Here's how the part is built. I have some questions about the finished solid (model axes, mm). A direction names the side the tool comes from. Give positions to 0.01 mm unless a question says otherwise; leave off trailing zeros. Order: outer loops, then holes, each group sorted by start corner. A loop starts at its lowest first (then second) coordinate and runs counter-clockwise, first axis right, second up. Notation, with made-up numbers: M 42,-19.75 L 66,-19.75 A19 ccw 66,0.25 Z; hole C 67,77 d11. An arc over 180 degrees is marked long. Use one line per item in the form item = value.
from build123d import *

# Parameters (mm, degrees)
F1_DEPTH  = 5
F0_W      = 15
F0_H      = 3
F2_DEPTH  = 15
F0_W_2    = 3
F3_DEPTH  = 3
F4_DEPTH  = 12
F6_DEPTH  = 25
F10_W     = 5
F10_H     = 5
F11_DEPTH = 2
F12_DEPTH = 12
F13_DEPTH = 9
F14_DEPTH = 6
F15_DEPTH = 9
F16_DEPTH = 9
F17_DEPTH = 15
F18_DEPTH = 12
F19_DEPTH = 6
F20_DEPTH = 9
F21_DEPTH = 12
F22_DEPTH = 9
F23_DEPTH = 3
F24_DEPTH = 4
F25_DEPTH = 6
F26_DEPTH = 1
F27_DEPTH = 3
F28_DEPTH = 5
F9_W      = 3
F9_H      = 3
F29_DEPTH = 2
F30_DEPTH = 4
F31_DEPTH = 6
F32_DEPTH = 8
F33_DEPTH = 1
F34_DEPTH = 3
F35_DEPTH = 5
F36_DEPTH = 7
F37_DEPTH = 1
F38_DEPTH = 2
F39_DEPTH = 3
F40_DEPTH = 4
F42_DEPTH = 3
F44_DEPTH = 3


with BuildPart() as f1:
    # F0 (on Top) → F1 (new body)
    with BuildSketch(Plane.XY):
        Polygon((14.2212225916, -3.3255452978), (14.1498658388, 11.6744547022), (-0.7787774084, 11.6744547022), (-0.7787774084, -3.3255452978), align=None)
    extrude(amount=F1_DEPTH)



with BuildPart() as f2:
    # F0 (on Top) → F2 (new body)
    with BuildSketch(Plane.XY):
        with Locations((-11.4361313693, -1.8255452978)):
            Rectangle(F0_W, F0_H)
    extrude(amount=F2_DEPTH)


with BuildPart() as f3:
    # F0 (on Top) → F3 (new body)
    with BuildSketch(Plane.XY):
        with Locations((-5.4361313693, 28.1744547022)):
            Rectangle(F0_W_2, F0_H)
    extrude(amount=F3_DEPTH)


with BuildPart() as f4:
    # F0 (on Top) → F4 (new body)
    with BuildSketch(Plane.XY):
        Polygon((2.0638686307, 29.6744547022), (-0.9361313693, 29.6744547022), (-0.9361313693, 14.7520447022), (-0.9361313693, 14.6744547022), (2.0638686307, 14.6744547022), (2.0638686307, 14.7520447022), align=None)
    extrude(amount=F4_DEPTH)


with BuildPart() as f1_1:
    add(f1.part)

    add(f2.part)  # F6 merges F2

    add(f3.part)  # F6 merges F3

    add(f4.part)  # F6 merges F4
    # F5 (on Top) → F6 (join)
    with BuildSketch(Plane.XY):
        Polygon((-18.9361313693, -3.3255452978), (14.2212225916, -3.3255452978), (14.0638686307, 29.7520447022), (-18.9361313693, 29.6744547022), align=None)
    extrude(amount=-F6_DEPTH)

    # F7 (on face) → F8 (revolve, cut)
    with BuildSketch(Plane.XZ.offset(3.3255452978)):
        with BuildLine():
            Line((-2.1231973078, -23.52852803), (-2.1231973078, -2.4096941548))
            ThreePointArc((-2.1231973078, -2.4096941548), (-12.6826142454, -12.9691110924), (-2.1231973078, -23.52852803))
        make_face()
    revolve(axis=Axis((-2.1231973078, -3.3255452978, -12.9691110924), (0, 0, -1)), mode=Mode.SUBTRACT)

    # F10 (on face) → F11 (cut)
    with BuildSketch(Plane(origin=(14.2050811207, 0.0675752308, 0), x_dir=(-0.004757063, 0.9999886851, 0), z_dir=(0.9999886851, 0.004757063, 0))):
        with Locations((2.0033325977, -6.7919711024)):
            Rectangle(F10_W, F10_H)
    extrude(amount=-F11_DEPTH, mode=Mode.SUBTRACT)

    # F0 (on Top) → F12 (join)
    with BuildSketch(Plane.XY):
        with Locations((-11.4361313693, 4.1744547022)):
            Rectangle(F0_W, F0_H)
    extrude(amount=F12_DEPTH)

    # F0 (on Top) → F13 (join)
    with BuildSketch(Plane.XY):
        with Locations((-11.4361313693, 10.1744547022)):
            Rectangle(F0_W, F0_H)
    extrude(amount=F13_DEPTH)

    # F0 (on Top) → F14 (join)
    with BuildSketch(Plane.XY):
        with Locations((-11.4361313693, 28.1744547022)):
            Rectangle(F0_W_2, F0_H)
    extrude(amount=F14_DEPTH)

    # F0 (on Top) → F15 (join)
    with BuildSketch(Plane.XY):
        with Locations((-17.4361313693, 28.1744547022)):
            Rectangle(F0_W_2, F0_H)
    extrude(amount=F15_DEPTH)

    # F0 (on Top) → F16 (join)
    with BuildSketch(Plane.XY):
        with Locations((-11.4361313693, 22.1744547022)):
            Rectangle(F0_W_2, F0_H)
    extrude(amount=F16_DEPTH)

    # F0 (on Top) → F17 (join)
    with BuildSketch(Plane.XY):
        with Locations((-17.4361313693, 16.1744547022)):
            Rectangle(F0_W_2, F0_H)
    extrude(amount=F17_DEPTH)

    # F0 (on Top) → F18 (join)
    with BuildSketch(Plane.XY):
        with Locations((-17.4361313693, 22.1744547022)):
            Rectangle(F0_W_2, F0_H)
    extrude(amount=F18_DEPTH)

    # F0 (on Top) → F19 (join)
    with BuildSketch(Plane.XY):
        with Locations((-5.4361313693, 22.1744547022)):
            Rectangle(F0_W_2, F0_H)
    extrude(amount=F19_DEPTH)

    # F0 (on Top) → F20 (join)
    with BuildSketch(Plane.XY):
        with Locations((-5.4361313693, 16.1744547022)):
            Rectangle(F0_W_2, F0_H)
    extrude(amount=F20_DEPTH)

    # F0 (on Top) → F21 (join)
    with BuildSketch(Plane.XY):
        with Locations((-11.4361313693, 16.1744547022)):
            Rectangle(F0_W_2, F0_H)
    extrude(amount=F21_DEPTH)

    # F0 (on Top) → F22 (join)
    with BuildSketch(Plane.XY):
        Polygon((8.0638686307, 29.6744547022), (5.0638686307, 29.6744547022), (5.0638686307, 14.7520447022), (5.0638686307, 14.6744547022), (8.0638686307, 14.6744547022), (8.0638686307, 14.7520447022), align=None)
    extrude(amount=F22_DEPTH)

    # F0 (on Top) → F23 (join)
    with BuildSketch(Plane.XY):
        Polygon((14.0638686307, 29.6744547022), (11.0638686307, 29.6744547022), (11.0638686307, 14.7520447022), (11.0638686307, 14.6744547022), (14.0638686307, 14.6744547022), (14.0638686307, 14.7520447022), align=None)
    extrude(amount=F23_DEPTH)

    # F10 (on face) → F24 (cut)
    with BuildSketch(Plane(origin=(14.2050811207, 0.0675752308, 0), x_dir=(-0.004757063, 0.9999886851, 0), z_dir=(0.9999886851, 0.004757063, 0))):
        with Locations((12.0033325977, -6.7919711024)):
            Rectangle(F10_W, F10_H)
    extrude(amount=-F24_DEPTH, mode=Mode.SUBTRACT)

    # F10 (on face) → F25 (cut)
    with BuildSketch(Plane(origin=(14.2050811207, 0.0675752308, 0), x_dir=(-0.004757063, 0.9999886851, 0), z_dir=(0.9999886851, 0.004757063, 0))):
        with Locations((22.0033325977, -6.7919711024)):
            Rectangle(F10_W, F10_H)
    extrude(amount=-F25_DEPTH, mode=Mode.SUBTRACT)

    # F10 (on face) → F26 (cut)
    with BuildSketch(Plane(origin=(14.2050811207, 0.0675752308, 0), x_dir=(-0.004757063, 0.9999886851, 0), z_dir=(0.9999886851, 0.004757063, 0))):
        with Locations((2.0033325977, -16.7919711024)):
            Rectangle(F10_W, F10_H)
    extrude(amount=-F26_DEPTH, mode=Mode.SUBTRACT)

    # F10 (on face) → F27 (cut)
    with BuildSketch(Plane(origin=(14.2050811207, 0.0675752308, 0), x_dir=(-0.004757063, 0.9999886851, 0), z_dir=(0.9999886851, 0.004757063, 0))):
        with Locations((12.0033325977, -16.7919711024)):
            Rectangle(F10_W, F10_H)
    extrude(amount=-F27_DEPTH, mode=Mode.SUBTRACT)

    # F10 (on face) → F28 (cut)
    with BuildSketch(Plane(origin=(14.2050811207, 0.0675752308, 0), x_dir=(-0.004757063, 0.9999886851, 0), z_dir=(0.9999886851, 0.004757063, 0))):
        with Locations((22.0033325977, -16.7919711024)):
            Rectangle(F10_W, F10_H)
    extrude(amount=-F28_DEPTH, mode=Mode.SUBTRACT)

    # F9 (on face) → F29 (cut)
    with BuildSketch(Plane(origin=(-18.9361313693, 0, 0), x_dir=(0, -1, 0), z_dir=(-1, 0, 0))):
        with Locations((-23.521638004, -6.4509857927)):
            Rectangle(F9_W, F9_H)
    extrude(amount=-F29_DEPTH, mode=Mode.SUBTRACT)

    # F9 (on face) → F30 (cut)
    with BuildSketch(Plane(origin=(-18.9361313693, 0, 0), x_dir=(0, -1, 0), z_dir=(-1, 0, 0))):
        with Locations((-17.521638004, -6.4509857927)):
            Rectangle(F9_W, F9_H)
    extrude(amount=-F30_DEPTH, mode=Mode.SUBTRACT)

    # F9 (on face) → F31 (cut)
    with BuildSketch(Plane(origin=(-18.9361313693, 0, 0), x_dir=(0, -1, 0), z_dir=(-1, 0, 0))):
        with Locations((-11.521638004, -6.4509857927)):
            Rectangle(F9_W, F9_H)
    extrude(amount=-F31_DEPTH, mode=Mode.SUBTRACT)

    # F9 (on face) → F32 (cut)
    with BuildSketch(Plane(origin=(-18.9361313693, 0, 0), x_dir=(0, -1, 0), z_dir=(-1, 0, 0))):
        with Locations((-5.521638004, -6.4509857927)):
            Rectangle(F9_W, F9_H)
    extrude(amount=-F32_DEPTH, mode=Mode.SUBTRACT)

    # F9 (on face) → F33 (cut)
    with BuildSketch(Plane(origin=(-18.9361313693, 0, 0), x_dir=(0, -1, 0), z_dir=(-1, 0, 0))):
        with Locations((-23.521638004, -12.4509857927)):
            Rectangle(F9_W, F9_H)
    extrude(amount=-F33_DEPTH, mode=Mode.SUBTRACT)

    # F9 (on face) → F34 (cut)
    with BuildSketch(Plane(origin=(-18.9361313693, 0, 0), x_dir=(0, -1, 0), z_dir=(-1, 0, 0))):
        with Locations((-17.521638004, -12.4509857927)):
            Rectangle(F9_W, F9_H)
    extrude(amount=-F34_DEPTH, mode=Mode.SUBTRACT)

    # F9 (on face) → F35 (cut)
    with BuildSketch(Plane(origin=(-18.9361313693, 0, 0), x_dir=(0, -1, 0), z_dir=(-1, 0, 0))):
        with Locations((-11.521638004, -12.4509857927)):
            Rectangle(F9_W, F9_H)
    extrude(amount=-F35_DEPTH, mode=Mode.SUBTRACT)

    # F9 (on face) → F36 (cut)
    with BuildSketch(Plane(origin=(-18.9361313693, 0, 0), x_dir=(0, -1, 0), z_dir=(-1, 0, 0))):
        with Locations((-5.521638004, -12.4509857927)):
            Rectangle(F9_W, F9_H)
    extrude(amount=-F36_DEPTH, mode=Mode.SUBTRACT)

    # F9 (on face) → F37 (cut)
    with BuildSketch(Plane(origin=(-18.9361313693, 0, 0), x_dir=(0, -1, 0), z_dir=(-1, 0, 0))):
        with Locations((-23.521638004, -18.4509857927)):
            Rectangle(F9_W, F9_H)
    extrude(amount=-F37_DEPTH, mode=Mode.SUBTRACT)

    # F9 (on face) → F38 (cut)
    with BuildSketch(Plane(origin=(-18.9361313693, 0, 0), x_dir=(0, -1, 0), z_dir=(-1, 0, 0))):
        with Locations((-17.521638004, -18.4509857927)):
            Rectangle(F9_W, F9_H)
    extrude(amount=-F38_DEPTH, mode=Mode.SUBTRACT)

    # F9 (on face) → F39 (cut)
    with BuildSketch(Plane(origin=(-18.9361313693, 0, 0), x_dir=(0, -1, 0), z_dir=(-1, 0, 0))):
        with Locations((-11.521638004, -18.4509857927)):
            Rectangle(F9_W, F9_H)
    extrude(amount=-F39_DEPTH, mode=Mode.SUBTRACT)

    # F9 (on face) → F40 (cut)
    with BuildSketch(Plane(origin=(-18.9361313693, 0, 0), x_dir=(0, -1, 0), z_dir=(-1, 0, 0))):
        with Locations((-5.521638004, -18.4509857927)):
            Rectangle(F9_W, F9_H)
    extrude(amount=-F40_DEPTH, mode=Mode.SUBTRACT)

    # F41 (on face) → F42 (join)
    with BuildSketch(Plane.XY.offset(5)):
        Polygon((-0.7787774084, -3.3255452978), (3.3940772992, -3.3255452978), (6.7212225916, 11.6744547022), (-0.7787774084, 11.6744547022), align=None)
    extrude(amount=F42_DEPTH)

    # F43 (on face) → F44 (join)
    with BuildSketch(Plane(origin=(-0.069875234, 29.7188132724, 0), x_dir=(-0.9999972359, -0.0023512056, 0), z_dir=(-0.0023512056, 0.9999972359, 0))):
        Polygon((18.8663082835, 0), (9.8840193823, 0), (-5.0577260554, -25), (18.8663082835, -25), align=None)
    extrude(amount=F44_DEPTH)


solid = f1_1.part
Q1. I want a section at B-B on z = -3.5. Write out the boundary of the cut face in (x, y), then the cut area to 3 significant figures.
Found:
outline = M -18.94,-3.33 L -6.8,-3.33 A4.67 cw 2.55,-3.33 L 14.22,-3.33 L 14.06,29.75 L -7.86,29.7 L -7.87,32.7 L -18.94,32.67 L -18.94,29.67 Z
area = 1,090 mm²
Q2. I want a section at D-D on x = 1.5. Write out the boundary of the cut face in (y, z).
Found:
outline = M -3.33,-25 L 32.72,-25 L 32.72,-19.18 L 29.72,-19.16 L 29.72,0 L 29.67,0 L 29.67,12 L 14.67,12 L 14.67,0 L 11.67,0 L 11.67,8 L -3.33,8 L -3.33,-3.05 A9.92 cw -3.33,-22.89 Z
Q3. On a 3-axis mill with a long thin cutter (end or side, diameter ignored), from which of +Z, -Z, +X, -X, +Y, -Y can I reach the whole of each face in a straight line? I mean faces 1 (the face through (-15, 6, -13.951)), 2 (the face through (-11, 14.674, 6)), 3 (the face through (12, 12, -4.292)). Say none if no direction works.
Found:
face_1 = -X
face_2 = +Z, +X, -X
face_3 = +X
Q4. I need wall thicknesses on L1, parallel to X at y = 17, z = 1; L2, parallel to Z at x = 10.5, y = 23; L3, parallel to X at y = 23.5, z = 7.5. Which ranges of each line are inside material? Lowest first, please.
Found:
L1 = -18.94 to -15.94, -12.94 to -9.94, -6.94 to -3.94, -0.94 to 2.06, 5.06 to 8.06, 11.06 to 14.06
L2 = -25 to -19.29, -14.29 to -9.29, -4.29 to 0
L3 = -18.94 to -15.94, -12.94 to -9.94, -0.94 to 2.06, 5.06 to 8.06
Q5. Thinking about a two-plate mould opening in Z: for faces 4 (the face through (-17, 10.022, -18)), 5 (the face through (7, 29.674, 4)), 6 (the face through (-11, 16, 12)), which applies, +Z half, -Z half, draft (parallel to the pull), parting line (faces both ways), or undercut?
Found:
face_4 = undercut
face_5 = draft
face_6 = +Z half
Q6. I'm going to push flat-ended pins straight in: pin 1 Ø1.5 at (x, y) = (-12, 15.5) entering from +Z; pin 2 Ø3.5 at (x, z) = (-15.5, -13) entering from +Y; pin 3 Ø3 at (x, z) = (8.5, -20) entering from +Y; pin 4 Ø6 at (x, y) = (-8.5, 2) entering from +Z. Where does each tip first touch, or does it pass through?
Found:
pin_1 = 12
pin_2 = 32.69
pin_3 = 29.74
pin_4 = 15
Q7. I want a section at C-C on y = 1. Write out the boundary of the cut face in (x, z).
Found:
outline = M -18.94,-25 L 14.2,-25 L 14.2,-19.29 L 13.2,-19.29 L 13.2,-14.29 L 14.2,-14.29 L 14.2,-9.29 L 12.2,-9.29 L 12.2,-4.29 L 14.2,-4.29 L 14.2,5 L 4.35,5 L 4.35,8 L -0.78,8 L -0.78,0 L -18.94,0 Z; hole C -2.12,-12.97 d19.27
